Source: CAD feature listing. Evaluate the final solid. Frame: model axes, mm. Face numbers are marked on the shaded views. A direction names the side the tool comes from. Round coordinates to 2 decimals unless told otherwise and drop trailing zeros. Loops run counter-clockwise (first coordinate to the right, second up) from the corner with the lowest first, then second, coordinate; pieces in that order, holes last.
(1) Mould query, pull axis X, two halves, no side actions, for the marked faces 4, 5, 6 and 7. Classes: pulls with the +X half, pulls with the -X half, needs draft (parallel to the pull), parting line crosses it, or undercut.
(2) First-contact query: pin 1 Ø4 at (x, z) = (11, 14.5) entering from -Y; pin 2 Ø1.5 at (x, y) = (24, 22) entering from -Z; pin 3 Ø1.5 at (x, y) = (27.5, 29) entering from +Z; pin 4 Ø1.5 at (x, z) = (22.5, 18) entering from +Y. Flat tips, straight axial feed; report the tip coordinate or a pass-through.
(3) Section B-B, the plane x = 18. Return the cut outline in (y, z), plus the area to 3 significant figures.
(4) Section C-C, the plane y = 33. Return the cut outline in (x, z), plus the area to 3 significant figures.
(5) Material intervals for probe 1 along Z at (x, y) = (18, 31); probe 2 along X at (y, z) = (30, 20); probe 3 along Z at (x, y) = (32.5, 23), sorted ascending.
(6) Set-up query: the marked faces 1, 2 and 3. Return all of +Z, -Z, +X, -X, +Y, -Y with unobstructed straight access to the full face (end or side cutting, diameter ignored); none if empty.
(7) Section D-D, the plane x = 5. Return the cut outline in (y, z).
(8) Section A-A, the plane z = 18.5. Return the cut outline in (x, y).
```python
from build123d import *

# Parameters (mm, degrees)
SKETCH1_W           = 38
SKETCH1_H           = 36
BOSS_EXTRUDE1_DEPTH = 5.5
SKETCH5_W           = 38
SKETCH5_H           = 5.5
BOSS_EXTRUDE5_DEPTH = 32.5
BOSS_EXTRUDE6_DEPTH = 3.4
BOSS_EXTRUDE7_DEPTH = 3.4
SKETCH9_W           = 8.9
SKETCH9_H           = 20
CUT_EXTRUDE1_DEPTH  = 62.791989772
FILLET1_R           = 1
CUT_EXTRUDE3_START  = -3
CUT_EXTRUDE3_DEPTH  = 3
SKETCH19_W          = 8.460607986
SKETCH19_H          = 6
CUT_EXTRUDE4_DEPTH  = 3


# Read off the part's stored shape, not the designer's step: Cut-Extrude3
with BuildPart() as part:
    # Sketch1 → Boss-Extrude1 (new body)
    with BuildSketch(Plane.XY):
        with Locations((19, 18)):
            Rectangle(SKETCH1_W, SKETCH1_H)
    extrude(amount=BOSS_EXTRUDE1_DEPTH)

    # Sketch5 → Boss-Extrude5 (add)
    with BuildSketch(Plane.XY.offset(5.5)):
        with Locations((19, 33.25)):
            Rectangle(SKETCH5_W, SKETCH5_H)
    extrude(amount=BOSS_EXTRUDE5_DEPTH)

    # Sketch7 → Boss-Extrude6 (add)
    with BuildSketch(Plane.ZY):
        Polygon((5.5, 0), (38, 30.5), (5.5, 30.5), align=None)
    extrude(amount=-BOSS_EXTRUDE6_DEPTH)

    # Sketch8 → Boss-Extrude7 (add)
    with BuildSketch(Plane(origin=(38, 0, 0), x_dir=(0, 0, -1), z_dir=(1, 0, 0))):
        Polygon((-5.5, 0), (-5.5, 30.5), (-38, 30.5), align=None)
    extrude(amount=-BOSS_EXTRUDE7_DEPTH)

    # Sketch9 → Cut-Extrude1 (cut, through all)
    with BuildSketch(Plane(origin=(0, 30.5, 0), x_dir=(-1, 0, 0), z_dir=(0, -1, 0))):
        with Locations((-19, -22.5)):
            Rectangle(SKETCH9_W, SKETCH9_H)
    extrude(amount=-CUT_EXTRUDE1_DEPTH, mode=Mode.SUBTRACT)

    # Fillet1
    fillet1_edges = [part.edges().sort_by_distance(p)[0] for p in [
        (23.45, 33.25, 32.5),
        (23.45, 33.25, 12.5),
        (14.55, 33.25, 12.5),
        (14.55, 33.25, 32.5),
    ]]
    fillet(fillet1_edges, radius=FILLET1_R)

    # Cut-Extrude3 outline → Cut-Extrude3 (cut)
    with BuildSketch(Plane(origin=(0, 0, 0), x_dir=(-1, 0, 0), z_dir=(0, 0, -1)).offset(CUT_EXTRUDE3_START)):
        with BuildLine():
            Line((-27.5, 21.122498999), (-27.5, 14.877501001))
            ThreePointArc((-27.5, 14.877501001), (-8, 18), (-27.5, 21.122498999))
        make_face()
    extrude(amount=CUT_EXTRUDE3_DEPTH, mode=Mode.SUBTRACT)

    # Sketch19 → Cut-Extrude4 (cut)
    with BuildSketch(Plane(origin=(0, 0, 0), x_dir=(-1, 0, 0), z_dir=(0, 0, -1))):
        with Locations((-4.230303993, 18)):
            Rectangle(SKETCH19_W, SKETCH19_H)
    extrude(amount=-CUT_EXTRUDE4_DEPTH, mode=Mode.SUBTRACT)


solid = part.part
```
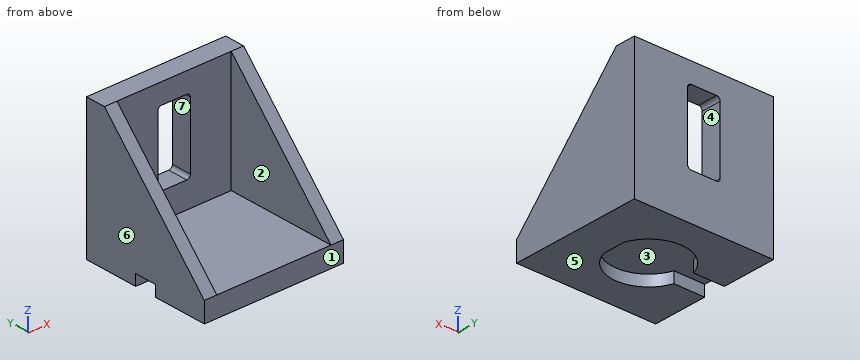
Output values:
1. face 4: undercut
1. face 5: needs draft
1. face 6: pulls with the -X half
1. face 7: undercut
2. pin 1: stops at y = 30.5
2. pin 2: stops at z = 3
2. pin 3: stops at z = 5.5
2. pin 4: passes through
3. outline: (0, 0) - (8, 0) - (8, 3) - (28, 3) - (28, 0) - (36, 0) - (36, 12.5) - (30.5, 12.5) - (30.5, 5.5) - (0, 5.5) - close; (30.5, 32.5) - (36, 32.5) - (36, 38) - (30.5, 38) - close
3. area: 207 mm2
4. outline: (0, 0) - (38, 0) - (38, 38) - (0, 38) - close; hole (14.55, 13.5) arc R1 ccw to (15.55, 12.5) - (22.45, 12.5) arc R1 ccw to (23.45, 13.5) - (23.45, 31.5) arc R1 ccw to (22.45, 32.5) - (15.55, 32.5) arc R1 ccw to (14.55, 31.5) - close
4. area: 1,270 mm2
5. probe 1: z = 0 to 12.5, 32.5 to 38
5. probe 2: x = 0 to 3.4, 34.6 to 38
5. probe 3: z = 0 to 5.5
6. face 1: +Z, -Z, +X, -X, -Y
6. face 2: +Z, -Y
6. face 3: -Z
7. outline: (0, 0) - (15, 0) - (15, 3) - (21, 3) - (21, 0) - (36, 0) - (36, 38) - (30.5, 38) - (30.5, 5.5) - (0, 5.5) - close
8. outline: (0, 12.2) - (3.4, 12.2) - (3.4, 30.5) - (14.55, 30.5) - (14.55, 36) - (0, 36) - close; (23.45, 30.5) - (34.6, 30.5) - (34.6, 12.2) - (38, 12.2) - (38, 36) - (23.45, 36) - close
